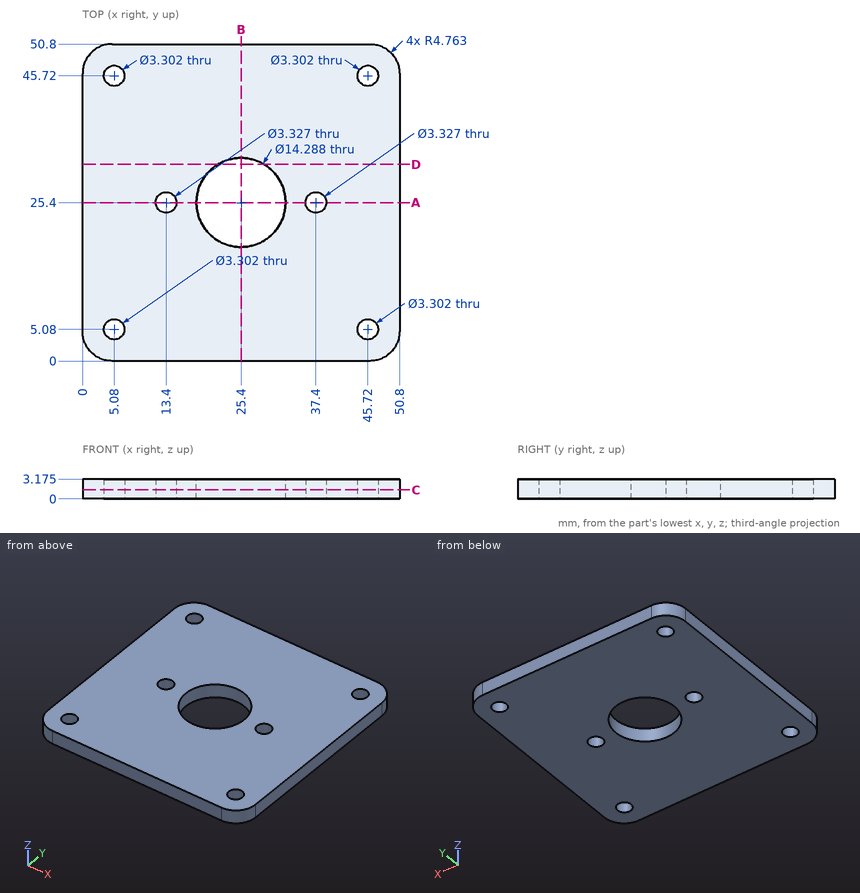
Geometry check sheet. Reference: drawing and pictorial views, mm from the part's lowest x, y, z. Coordinates: 2 decimals unless noted, no trailing zeros. Order: outer loops, then holes, each group sorted by start corner. A loop starts at its lowest first (then second) coordinate and runs counter-clockwise, first axis right, second up. Notation, with made-up numbers: (-17, -32) -> (-12, -32) arc R14 cw to (-12, -11) -> close; hole circle Ø4 at (-25.75, -15.5). An arc over 180 degrees is marked (long way). Put each result on its own line as item: value. Start each with the question number.
1) Cross-section at A-A (y = 25.4). Enter the section's corners in (x, z) (1 decimal).
2) Cross-section at B-B (x = 25.4). Enter the section's corners in (y, z) (1 decimal), plus the area to 3 significant figures.
3) Cross-section at D-D (y = 31.5). Enter the section's corners in (x, z) (1 decimal).
4) Material ranges on L1, parallel to X at y = 45.72, z = 0.65; L2, parallel to Y at x = 45.5, z = 2.9 (1 decimal); L3, parallel to Y at x = 25.4, z = 1.25, recorded low to high.
5) Cross-section at C-C (z = 1.45). State how many separate pieces and enclosed holes the cut face has, plus the area to 3 significant figures.
Geometry check:
1. outline: (0, 0) -> (11.7, 0) -> (11.7, 3.2) -> (0, 3.2) -> close; (15.1, 0) -> (18.3, 0) -> (18.3, 3.2) -> (15.1, 3.2) -> close; (32.5, 0) -> (35.7, 0) -> (35.7, 3.2) -> (32.5, 3.2) -> close; (39.1, 0) -> (50.8, 0) -> (50.8, 3.2) -> (39.1, 3.2) -> close
2. outline: (0, 0) -> (18.3, 0) -> (18.3, 3.2) -> (0, 3.2) -> close; (32.5, 0) -> (50.8, 0) -> (50.8, 3.2) -> (32.5, 3.2) -> close
2. area: 116 mm^2
3. outline: (0, 0) -> (21.7, 0) -> (21.7, 3.2) -> (0, 3.2) -> close; (29.1, 0) -> (50.8, 0) -> (50.8, 3.2) -> (29.1, 3.2) -> close
4. L1: x = 0 to 3.43, 6.73 to 44.07, 47.37 to 50.8
4. L2: y = 0 to 3.4, 6.7 to 44.1, 47.4 to 50.8
4. L3: y = 0 to 18.26, 32.54 to 50.8
5. separate pieces: 1
5. enclosed holes: 7
5. area: 2,350 mm^2
